```python
from build123d import *

# Parameters (mm, degrees)
F0_W     = 76.2
F0_H     = 98.425
F1_DEPTH = 3.175
F2_W     = 12.7
F2_H     = 3.175
F3_DEPTH = 3.176
F4_W     = 3.175
F4_H     = 12.7
F5_DEPTH = 3.176
F7_DEPTH = 3.176


with BuildPart() as f1:
    # F0 (on Front) → F1 (new body)
    with BuildSketch(Plane.XZ):
        Rectangle(F0_W, F0_H)
    extrude(amount=F1_DEPTH)

    # F2 (on face) → F3 (cut, through all)
    with BuildSketch(Plane.XZ.offset(3.175)):
        with Locations((-31.75, 47.625)):
            Rectangle(F2_W, F2_H)
        with Locations((0, 47.625)):
            Rectangle(F2_W, F2_H)
        with Locations((31.75, 47.625)):
            Rectangle(F2_W, F2_H)
    extrude(amount=-F3_DEPTH, mode=Mode.SUBTRACT)

    # F4 (on face) → F5 (cut, through all)
    with BuildSketch(Plane.XZ.offset(3.175)):
        with Locations((-36.5125, 42.8625)):
            Rectangle(F4_W, F4_H)
        with Locations((-36.5125, 14.2875)):
            Rectangle(F4_W, F4_H)
        with Locations((-36.5125, -14.2875)):
            Rectangle(F4_W, F4_H)
        with Locations((-36.5125, -42.8625)):
            Rectangle(F4_W, F4_H)
        with Locations((36.5125, -42.8625)):
            Rectangle(F4_W, F4_H)
        with Locations((36.5125, 14.2875)):
            Rectangle(F4_W, F4_H)
        with Locations((36.5125, -14.2875)):
            Rectangle(F4_W, F4_H)
        with Locations((36.5125, 42.8625)):
            Rectangle(F4_W, F4_H)
    extrude(amount=-F5_DEPTH, mode=Mode.SUBTRACT)

    # F6 (on face) → F7 (cut, through all)
    with BuildSketch(Plane.XZ.offset(3.175)):
        with BuildLine():
            add(Edge.make_bspline(
                [(15.875, -49.2125), (15.875, -21.716193), (-7.9375, -35.464347), (-31.75, -49.2125), (-7.9375, -62.960653), (15.875, -76.708807), (15.875, -49.2125)],
                knots=[0, 0, 0, 2.094395, 2.094395, 4.18879, 4.18879, 6.283185, 6.283185, 6.283185], degree=2, weights=[1, 0.5, 1, 0.5, 1, 0.5, 1]))
        make_face()
    extrude(amount=-F7_DEPTH, mode=Mode.SUBTRACT)


solid = f1.part
```
The model under review builds one solid part; all positions refer to its coordinate system, in mm. A direction names the side the tool comes from. Coordinates: 2 decimals unless noted, no trailing zeros. Order: outer loops, then holes, each group sorted by start corner. A loop starts at its lowest first (then second) coordinate and runs counter-clockwise, first axis right, second up. Notation, with made-up numbers: (88.5, -28) -> (145.5, -28) arc R25 ccw to (145.5, -10) -> close; hole circle Ø8 at (11.25, 13.5). An arc over 180 degrees is marked (long way). Answer in a Markdown table with one row per item. Add a question column.
Item 1: Clearance check with flat-ended pins moving along their axes: pin 1 (1 mm diameter, centred on x = -36, y = -1, fed in from +Z); pin 2 (1.6 mm diameter, centred on y = -1, z = 48, fed in from -X); pin 3 (1 mm diameter, centred on y = -1.5, z = 47.5, fed in from +X). State where each tip first meets the part, or that it passes through.
Item 2: We need section A-A on z = -9.5. Write out the cut boundary in (x, y) (3 decimals).
Item 3: To check wall thickness, follow probe 1 along Z at (x, y) = (33, -0.6); probe 2 along X at (y, z) = (-1.5, -40.5) (3 decimals); probe 3 along X at (y, z) = (-2.3, -9) (3 decimals). State the ranges of each line that lie inside material, in increasing order.
Item 4: We need section B-B on x = 30.5. Write out the cut boundary in (y, z) (1 decimal), plus the area to 3 significant figures.
Item 5: Mouldability with a two-part tool opening along Z and no side actions: class faces 1 (the flat face through (-37, -2, -7.938)), 2 (the flat face through (-6.35, -2, 48)), 3 (the flat face through (-26, -2, -49.212)) as +Z half, -Z half, draft (parallel to the pull), parting line (faces both ways), or undercut.
Item 6: Machinability: for faces 4 (the flat face through (34.925, -2, -43)), 5 (the flat face through (34.925, -2, 41)), 6 (the flat face through (-30, -2, 46.038)), 7 (the flat face through (36, -2, -7.938)), 8 (the flat face through (-37, -2, -36.512)), which of the approach directions +Z, -Z, +X, -X, +Y, -Y give a long, thin tool a straight path to every point of the face, cutting with its end or side? Answer none if there is none.
Final values:
| question | item | result |
|---|---|---|
| 1 | pin 1 | stops at z = 36.51 |
| 1 | pin 2 | stops at x = -25.4 |
| 1 | pin 3 | stops at x = 25.4 |
| 2 | outline | (-34.925, -3.175) -> (34.925, -3.175) -> (34.925, 0) -> (-34.925, 0) -> close |
| 3 | probe 1 | z = -49.21 to 46.04 |
| 3 | probe 2 | x = -34.925 to -13.271, 13.271 to 34.925 |
| 3 | probe 3 | x = -34.925 to 34.925 |
| 4 | outline | (-3.2, -49.2) -> (0, -49.2) -> (0, 46) -> (-3.2, 46) -> close |
| 4 | area | 302 mm2 |
| 5 | face 1 | undercut |
| 5 | face 2 | draft |
| 5 | face 3 | -Z half |
| 6 | face 4 | -Z, +X, +Y, -Y |
| 6 | face 5 | +Z, +X, +Y, -Y |
| 6 | face 6 | +Z, -X, +Y, -Y |
| 6 | face 7 | +X, +Y, -Y |
| 6 | face 8 | -Z, -X, +Y, -Y |
